Can you work these out from the model? Positions are in its coordinate system, mm. A direction names the side the tool comes from. Coordinates: 2 decimals unless noted, no trailing zeros. Loops run counter-clockwise (first coordinate to the right, second up) from the corner with the lowest first, then second, coordinate; pieces in that order, holes last. Notation, with made-up numbers: (76, 2) - (96, 2) arc R22 cw to (96, 29) - close; hole circle Ø5 at (21, 80). An arc over 180 degrees is marked (long way). Put each result on its own line as item: value. Start each with the question number.
from build123d import *

# Parameters (mm, degrees)
F1_DEPTH = 152.4
F2_R     = 1.98374
F3_R     = 3.69316
F4_W     = 9.5329248
F4_H     = 24
F4_R     = 1.35255
F5_DEPTH = 1.70942
F6_W     = 24
F6_H     = 9.5329248
F6_R     = 1.35255
F7_DEPTH = 89.0613408
F8_W     = 6
F8_H     = 3.175
F9_DEPTH = 1.70942


with BuildPart() as f1:
    # F0 (on Top) → F1 (new body)
    with BuildSketch(Plane.XY):
        Polygon((0, 32.3337428), (0, 0), (-85.6425008, 0), (-85.6425008, 32.3337428), (-87.3519208, 32.3337428), (-87.3519208, -1.70942), (1.70942, -1.70942), (1.70942, 32.3337428), align=None)
    extrude(amount=F1_DEPTH)

    # F2
    f2_edges = [f1.edges().sort_by_distance(p)[0] for p in [
        (0, 0, 76.2),
        (-85.642501, 0, 76.2),
    ]]
    fillet(f2_edges, radius=F2_R)

    # F3
    f3_edges = [f1.edges().sort_by_distance(p)[0] for p in [
        (1.70942, -1.70942, 76.2),
        (-87.351921, -1.70942, 76.2),
    ]]
    fillet(f3_edges, radius=F3_R)

    # F4 (on face) → F5 (cut, through all)
    with BuildSketch(Plane(origin=(0, 0, 0), x_dir=(-1, 0, 0), z_dir=(0, 1, 0))):
        with Locations((74.5712504, 15.175)):
            Rectangle(F4_W, F4_H)
        with Locations((11.0712504, 15.175)):
            Rectangle(F4_W, F4_H)
        with Locations((11.0712504, 137.225)):
            Rectangle(F4_W, F4_H)
        with Locations((74.5712504, 137.225)):
            Rectangle(F4_W, F4_H)
        with Locations((60.20308, 6.35)):
            Circle(F4_R)
        with Locations((25.4394208, 6.35)):
            Circle(F4_R)
        with Locations((25.4394208, 146.05)):
            Circle(F4_R)
        with Locations((60.20308, 146.05)):
            Circle(F4_R)
    extrude(amount=-F5_DEPTH, mode=Mode.SUBTRACT)

    # F6 (on face) → F7 (cut, through all)
    with BuildSketch(Plane(origin=(-87.3519208, 0, 0), x_dir=(0, -1, 0), z_dir=(-1, 0, 0))):
        with Locations((-17.15874, 31.6544706)):
            Rectangle(F6_W, F6_H)
        with Locations((-17.15874, 120.7455294)):
            Rectangle(F6_W, F6_H)
        with Locations((-25.98374, 46.022641)):
            Circle(F6_R)
        with Locations((-25.98374, 106.377359)):
            Circle(F6_R)
        with Locations((-8.33374, 106.377359)):
            Circle(F6_R)
        with Locations((-8.33374, 46.022641)):
            Circle(F6_R)
    extrude(amount=-F7_DEPTH, mode=Mode.SUBTRACT)

    # F8 (on face) → F9 (cut, through all)
    with BuildSketch(Plane.YZ.offset(1.70942)):
        with Locations((17.1587414, 4.7625)):
            Rectangle(F8_W, F8_H)
        with Locations((17.1587414, 147.6375)):
            Rectangle(F8_W, F8_H)
    extrude(amount=-F9_DEPTH, mode=Mode.SUBTRACT)


solid = f1.part
Q1. We'd pull the mould along Z, two halves only. Please class faces 1 (the flat face through (-43, -1.709, 75)), 2 (the flat face through (-63, -1, 152.4)), 3 (the cylindrical face through (-86.509, 27.057, 45.2)): released by +Z, released by -Z, zero draft, split by the parting line, or undercut.
Q2. I want a section at A-A on z = 29. List the corners of the cut face in (x, y) for me, and give its area (3 significant figures).
Q3. I want a section at C-C on x = -63. List the corners of the cut face in (y, z) for me.
Q4. I want a section at B-B on z = 76. List the corners of the cut face in (x, y) for me, and give its area (3 significant figures).
Q5. Will these pins go through, and if not, where does the flat tip stop? pin 1 (0.9 mm diameter, centred on x = 1, z = 33, fed in from -Y); pin 2 (0.9 mm diameter, centred on y = -0.5, z = 142, fed in from +X); pin 3 (0.9 mm diameter, centred on y = -1, z = 139.5, fed in from +X).
Q6. Please list where these lines run through material, in increasing order: line 1 along X through (y, z) = (23.5, 135.5); line 2 along X through (y, z) = (-1, 6); line 3 along Y through (x, z) = (-67, 14). Write a range as [from, to].
Q7. On a 3-axis mill with a long thin cutter (end or side, diameter ignored), from which of +Z, -Z, +X, -X, +Y, -Y can I reach the whole of each face in a straight line? I mean faces 4 (the flat face through (0, 17, 75)), 5 (the cylindrical face through (-86.509, 8.627, 44.702)). Say none if no direction works.
Calculated:
1. face 1: zero draft
1. face 2: released by +Z
1. face 3: undercut
2. outline: (-87.35, 1.98) arc R3.69 ccw to (-83.66, -1.71) - (-1.98, -1.71) arc R3.69 ccw to (1.71, 1.98) - (1.71, 5.16) - (0, 5.16) - (0, 1.98) arc R1.98 cw to (-1.98, 0) - (-83.66, 0) arc R1.98 cw to (-85.64, 1.98) - (-85.64, 5.16) - (-87.35, 5.16) - close; (-87.35, 29.16) - (-85.64, 29.16) - (-85.64, 32.33) - (-87.35, 32.33) - close; (0, 29.16) - (1.71, 29.16) - (1.71, 32.33) - (0, 32.33) - close
2. area: 177 mm2
3. outline: (-1.71, 0) - (0, 0) - (0, 152.4) - (-1.71, 152.4) - close
4. outline: (-87.35, 1.98) arc R3.69 ccw to (-83.66, -1.71) - (-1.98, -1.71) arc R3.69 ccw to (1.71, 1.98) - (1.71, 32.33) - (0, 32.33) - (0, 1.98) arc R1.98 cw to (-1.98, 0) - (-83.66, 0) arc R1.98 cw to (-85.64, 1.98) - (-85.64, 32.33) - (-87.35, 32.33) - close
4. area: 259 mm2
5. pin 1: y = -0.7
5. pin 2: x = 1.1
5. pin 3: x = 0.7
6. line 1: [-87.35, -85.64], [0, 1.71]
6. line 2: [-85.84, -79.34], [-69.8, -61.51], [-58.9, -26.75], [-24.13, -15.84], [-6.3, 0.19]
6. line 3: [-1.71, 0]
7. face 4: +Z, -Z, +Y
7. face 5: +X, -X
